The model under review builds one solid part; all positions refer to its coordinate system, in mm. Round coordinates to 2 decimals unless told otherwise and drop trailing zeros. Write each loop counter-clockwise with the first axis right and the second up, starting at its lowest first coordinate (ties: lowest second). Pieces come first, ordered by that corner, then holes. Notation, with made-up numbers: (8, 34.5) -> (67, 34.5) arc R8 cw to (67, 42.5) -> close; hole circle Ø5 at (74.5, 67). An arc over 180 degrees is marked (long way). Answer as a JSON object with one key per item and string values. Group by question number.
1) To check wall thickness, follow probe 1 along Y at (x, z) = (0, 0.95); probe 2 along X at (y, z) = (-3.5, 1.4); probe 3 along X at (y, z) = (-1.5, 1.1). State the ranges of each line that lie inside material, in increasing order. Write a range as [from, to].
2) We need section C-C, the plane y = -3.25. Write out the cut boundary in (x, z).
3) Mouldability with a two-part tool opening along X and no side actions: class faces 1 (the flat face through (-8, 6, 1)), 2 (the flat face through (-5.906, 9.122, 0.74)), 3 (the flat face through (5.96, 9.18, 0.74)), 4 (the flat face through (8, 6, 1)) as pulls with the +X half, pulls with the -X half, needs draft (parallel to the pull), parting line crosses it, or undercut.
4) We need section A-A, the plane z = 1.25. Write out the cut boundary in (x, y).
5) We need section B-B, the plane x = 0. Write out the cut boundary in (y, z), then the cut area to 3 significant figures.
6) Insertion check: pin 1 Ø1.5 at (x, y) = (1, 7) entering from -Z. The pin has a flat end and moves straight along its axis. Give the tip position at first contact, or say it passes through.
from build123d import *

# Parameters (mm, degrees)
F0_R     = 7
F1_DEPTH = 1.5


with BuildPart() as f1:
    # F0 (on Top) → F1 (new body)
    with BuildSketch(Plane.XY):
        with BuildLine():
            ThreePointArc((-8, 0), (0, -8), (8, 0))
            ThreePointArc((8, 0), (6.890506, 4.064594), (3.869769, 7.001777))
            ThreePointArc((3.869769, 7.001777), (0, 8), (-3.869769, 7.001777))
            ThreePointArc((-3.869769, 7.001777), (-6.890506, 4.064594), (-8, 0))
        make_face()
        Circle(F0_R, mode=Mode.SUBTRACT)
        with BuildLine():
            ThreePointArc((3.869769, 7.001777), (6.890506, 4.064594), (8, 0))
            Line((8, 0), (8, 11.303381))
            Line((8, 11.303381), (3.869769, 7.001777))
        make_face()
        with BuildLine():
            Line((-8, 11.303381), (-8, 0))
            ThreePointArc((-8, 0), (-6.890506, 4.064594), (-3.869769, 7.001777))
            Line((-3.869769, 7.001777), (-8, 11.303381))
        make_face()
    extrude(amount=F1_DEPTH)


solid = f1.part
Here are the results:
{
 "1": {"probe 1": "y = [-8, -7], [7, 8]", "probe 2": "x = [-7.19, -6.06], [6.06, 7.19]", "probe 3": "x = [-7.86, -6.84], [6.84, 7.86]"},
 "2": {"outline": "(-7.31, 0) -> (-6.2, 0) -> (-6.2, 1.5) -> (-7.31, 1.5) -> close; (6.2, 0) -> (7.31, 0) -> (7.31, 1.5) -> (6.2, 1.5) -> close"},
 "3": {"face 1": "pulls with the -X half", "face 2": "undercut", "face 3": "undercut", "face 4": "pulls with the +X half"},
 "4": {"outline": "(-8, 0) arc R8 ccw to (8, 0) -> (8, 11.3) -> (3.87, 7) arc R8 ccw to (-3.87, 7) -> (-8, 11.3) -> close; hole circle Ø14 at (0, 0)"},
 "5": {"outline": "(-8, 0) -> (-7, 0) -> (-7, 1.5) -> (-8, 1.5) -> close; (7, 0) -> (8, 0) -> (8, 1.5) -> (7, 1.5) -> close", "area": "3.00 mm^2"},
 "6": {"pin 1": "stops at z = 0"}
}
